from build123d import *

# Parameters (mm, degrees)
F0_R     = 60
F0_R_2   = 2.6
F1_DEPTH = 8
F2_R     = 2.6
F3_DEPTH = 5


with BuildPart() as f1:
    # F0 (on Top) → F1 (new body)
    with BuildSketch(Plane.XY):
        Circle(F0_R)
        with Locations((-32.5, 0)):
            Circle(F0_R_2, mode=Mode.SUBTRACT)
        with Locations((32.5, 0)):
            Circle(F0_R_2, mode=Mode.SUBTRACT)
    extrude(amount=F1_DEPTH)

    # F2 (on face) → F3 (cut)
    with BuildSketch(Plane.XY.offset(8)):
        Polygon((37.26314, 0), (34.88157, 4.125), (30.11843, 4.125), (27.73686, 0), (30.11843, -4.125), (34.88157, -4.125), align=None)
        with Locations((32.5, 0)):
            Circle(F2_R, mode=Mode.SUBTRACT)
        Polygon((-30.11843, 4.125), (-34.88157, 4.125), (-37.26314, 0), (-34.88157, -4.125), (-30.11843, -4.125), (-27.73686, 0), align=None)
        with Locations((-32.5, 0)):
            Circle(F2_R, mode=Mode.SUBTRACT)
    extrude(amount=-F3_DEPTH, mode=Mode.SUBTRACT)


solid = f1.part
Design review of the part built by this model. Coordinates are the model's own, in mm. A direction names the side the tool comes from. Round coordinates to 2 decimals unless told otherwise and drop trailing zeros. Loops run counter-clockwise (first coordinate to the right, second up) from the corner with the lowest first, then second, coordinate; pieces in that order, holes last. Notation, with made-up numbers: (31, 61.5) - (72, 61.5) arc R15 cw to (72, 81.5) - close; hole circle Ø6 at (-19.5, 12). An arc over 180 degrees is marked (long way). One line per question, with ' | ' between items.
1. For faces 4 (the face through (-33, -4.125, 6)), 5 (the face through (-1, 1, 8)), list the 3-axis set-ups (+Z, -Z, +X, -X, +Y, -Y) from which the entire face can be reached by the end or side of a thin tool; tool diameter is ignored.
Results are:
face 4: +Z | face 5: +Z, +X, -X, +Y, -Y
2. For L1, parallel to X at y = 1, z = 5.25; L2, parallel to X at y = 0.5, z = 1.25; L3, parallel to Y at x = 32.5, z = 1.1, list the stretches that pass through material, from the lowest coordinate up. Write a range as [from, to].
Results are:
L1: x = [-59.99, -36.69], [-28.31, 28.31], [36.69, 59.99] | L2: x = [-60, -35.05], [-29.95, 29.95], [35.05, 60] | L3: y = [-50.44, -2.6], [2.6, 50.44]
3. We need section A-A, the plane z = 6. State the section outline as (x, y) points (3 decimals), and give its area (3 significant figures).
Results are:
outline: circle Ø120 at (0, 0); hole (-37.263, 0) - (-34.882, -4.125) - (-30.118, -4.125) - (-27.737, 0) - (-30.118, 4.125) - (-34.882, 4.125) - close; hole (27.737, 0) - (30.118, -4.125) - (34.882, -4.125) - (37.263, 0) - (34.882, 4.125) - (30.118, 4.125) - close | area: 11,200 mm²
4. Clearance check with flat-ended pins moving along their axes: P1, Ø1.4, axis at x = 33, z = 5.5, coming from the -Y side; P2, Ø2.5, axis at x = -33.5, z = 5, coming from the +Y side; P3, Ø1, axis at x = -37.5, z = 6.5, coming from the -Y side; P4, Ø4, axis at x = 32.5, y = 0, coming from the -Z side. State where each tip first meets the part, or that it passes through.
Results are:
P1: stops at y = -50.56 | P2: stops at y = 50.6 | P3: stops at y = -47.23 | P4: passes through
5. We need section C-C, the plane y = 14.5. State the section outline as (x, z) points.
Results are:
outline: (-58.22, 0) - (58.22, 0) - (58.22, 8) - (-58.22, 8) - close
6. Draft analysis for pull direction X (two halves, no side actions). For faces 1 (the face through (-59.94, 2.64, 3.94)), 2 (the face through (-1, 1, 0)), 3 (the face through (-28.944, -2.091, 5.535)), state which applies: released by +X, released by -X, zero draft, split by the parting line, or undercut.
Results are:
face 1: split by the parting line | face 2: zero draft | face 3: undercut
7. We need section B-B, the plane x = -32.5. State the section outline as (y, z) points (3 decimals), and give its area (3 significant figures).
Results are:
outline: (-50.436, 0) - (-2.6, 0) - (-2.6, 3) - (-4.125, 3) - (-4.125, 8) - (-50.436, 8) - close; (2.6, 0) - (50.436, 0) - (50.436, 8) - (4.125, 8) - (4.125, 3) - (2.6, 3) - close | area: 750 mm²
8. We need section D-D, the plane x = 16. State the section outline as (y, z) points.
Results are:
outline: (-57.83, 0) - (57.83, 0) - (57.83, 8) - (-57.83, 8) - close
